from build123d import *

# Parameters (mm, degrees)
SKETCH1_R           = 5.05
BOSS_EXTRUDE1_DEPTH = 20
SKETCH2_R           = 9.25
CUT_EXTRUDE1_DEPTH  = 8
SKETCH4_R           = 7
SKETCH4_R_2         = 4
BOSS_EXTRUDE2_DEPTH = 2
CUT_EXTRUDE2_DEPTH  = 10


with BuildPart() as part:
    # Sketch1 → Boss-Extrude1 (new body)
    with BuildSketch(Plane.XY):
        with BuildLine():
            Line((-3, 10.5), (3, 10.5))
            Line((3, 10.5), (3, 11.618950039))
            ThreePointArc((3, 11.618950039), (8.485281374, 8.485281374), (11.618950039, 3))
            Line((11.618950039, 3), (10.5, 3))
            Line((10.5, 3), (10.5, -3))
            Line((10.5, -3), (11.618950039, -3))
            ThreePointArc((11.618950039, -3), (8.485281374, -8.485281374), (3, -11.618950039))
            Line((3, -11.618950039), (3, -10.5))
            Line((3, -10.5), (-3, -10.5))
            Line((-3, -10.5), (-3, -11.618950039))
            ThreePointArc((-3, -11.618950039), (-8.485281374, -8.485281374), (-11.618950039, -3))
            Line((-11.618950039, -3), (-10.5, -3))
            Line((-10.5, -3), (-10.5, 3))
            Line((-10.5, 3), (-11.618950039, 3))
            ThreePointArc((-11.618950039, 3), (-8.485281374, 8.485281374), (-3, 11.618950039))
            Line((-3, 11.618950039), (-3, 10.5))
        make_face()
        Circle(SKETCH1_R, mode=Mode.SUBTRACT)
    extrude(amount=BOSS_EXTRUDE1_DEPTH)

    # Sketch2 → Cut-Extrude1 (cut)
    with BuildSketch(Plane.XY.offset(20)):
        Circle(SKETCH2_R)
    extrude(amount=-CUT_EXTRUDE1_DEPTH, mode=Mode.SUBTRACT)

    # Cut-Sweep1: sweep along a curve in space
    with BuildLine() as cut_sweep1_path:
        ThreePointArc((9.25, 0, 20), (6.540737726, 6.540737726, 20), (0, 9.25, 20))
        ThreePointArc((0, 9.25, 20), (-6.540737726, 6.540737726, 20), (-9.25, 0, 20))
        ThreePointArc((-9.25, 0, 20), (-6.540737726, -6.540737726, 20), (0, -9.25, 20))
        ThreePointArc((0, -9.25, 20), (6.540737726, -6.540737726, 20), (9.25, 0, 20))
    # Sketch3 → Cut-Sweep1 (sweep, cut)
    with BuildSketch(Plane.XZ.offset(-3)):
        Polygon((10.118950039, 8.968340129), (10.118950039, 11.031659871), (11.618950039, 13.629736082), (11.618950039, 6.370263918), align=None)
    sweep(path=cut_sweep1_path.line, mode=Mode.SUBTRACT)

    # Sketch4 → Boss-Extrude2 (add)
    with BuildSketch(Plane.XY.offset(12)):
        Circle(SKETCH4_R)
        Circle(SKETCH4_R_2, mode=Mode.SUBTRACT)
    extrude(amount=-BOSS_EXTRUDE2_DEPTH)

    # Sketch5 → Cut-Extrude2 (cut)
    with BuildSketch(Plane(origin=(0, 0, 0), x_dir=(-1, 0, 0), z_dir=(0, 0, -1))):
        with BuildLine():
            Line((-11.618950039, 3), (-9.618950039, 3))
            ThreePointArc((-9.618950039, 3), (-8.204736476, 2.414213562), (-7.618950039, 1))
            Line((-7.618950039, 1), (-7.618950039, -1))
            ThreePointArc((-7.618950039, -1), (-8.204736476, -2.414213562), (-9.618950039, -3))
            Line((-9.618950039, -3), (-11.618950039, -3))
            Line((-11.618950039, -3), (-11.618950039, 3))
        make_face()
        with BuildLine():
            Line((-3, -11.618950039), (3, -11.618950039))
            Line((3, -11.618950039), (3, -9.618950039))
            ThreePointArc((3, -9.618950039), (2.414213562, -8.204736476), (1, -7.618950039))
            Line((1, -7.618950039), (-1, -7.618950039))
            ThreePointArc((-1, -7.618950039), (-2.414213562, -8.204736476), (-3, -9.618950039))
            Line((-3, -9.618950039), (-3, -11.618950039))
        make_face()
        with BuildLine():
            Line((3, 11.618950039), (3, 9.618950039))
            ThreePointArc((3, 9.618950039), (2.414213562, 8.204736476), (1, 7.618950039))
            Line((1, 7.618950039), (-1, 7.618950039))
            ThreePointArc((-1, 7.618950039), (-2.414213562, 8.204736476), (-3, 9.618950039))
            Line((-3, 9.618950039), (-3, 11.618950039))
            Line((-3, 11.618950039), (3, 11.618950039))
        make_face()
        with BuildLine():
            Line((11.618950039, -3), (9.618950039, -3))
            ThreePointArc((9.618950039, -3), (8.204736476, -2.414213562), (7.618950039, -1))
            Line((7.618950039, -1), (7.618950039, 1))
            ThreePointArc((7.618950039, 1), (8.204736476, 2.414213562), (9.618950039, 3))
            Line((9.618950039, 3), (11.618950039, 3))
            Line((11.618950039, 3), (11.618950039, -3))
        make_face()
    extrude(amount=-CUT_EXTRUDE2_DEPTH, mode=Mode.SUBTRACT)


solid = part.part
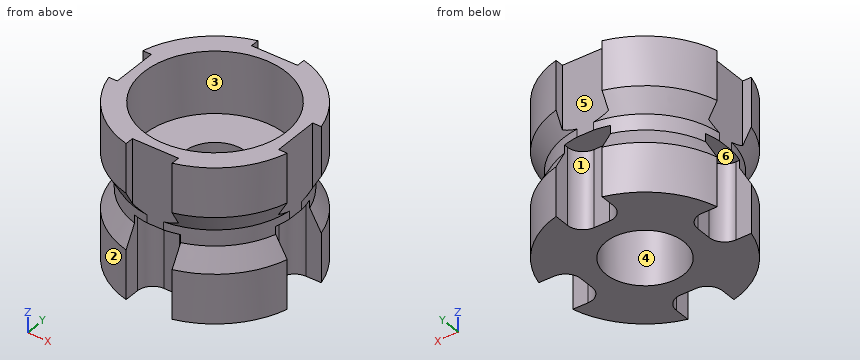
Check sheet for the modelled part. Datum: model origin and axes. Units: mm. Face numbers are marked on the shaded views. A direction names the side the tool comes from. Round coordinates to 2 decimals unless told otherwise and drop trailing zeros. Order: outer loops, then holes, each group sorted by start corner. A loop starts at its lowest first (then second) coordinate and runs counter-clockwise, first axis right, second up.
(1) Cross-section at D-D, the plane z = 10.5. Enter the section's corners in (x, y), and give its area (3 significant figures).
(2) Go/stop test with flat-tipped pins: P1, Ø0.9, axis at x = 11, z = 15.5, coming from the -Y side; P2, Ø1, axis at y = 11, z = 7, coming from the +X side; P3, Ø1, axis at y = -1.5, z = 18, coming from the -X side; P4, Ø8, axis at x = 1.5, y = -4.5, coming from the -Z side. Record where each tip stops, or that it passes through.
(3) Cross-section at A-A, the plane y = 0. Enter the section's corners in (x, z), and give its area (3 significant figures).
(4) Access from +Z, -Z, +X, -X, +Y, -Y to the whole of each face (thin tool, end or side, straight path). Record for the marked faces 4, 5 and 6.
(5) Scan lines: probe 1 along Y at (x, z) = (0, 10.9); probe 2 along Y at (x, z) = (0, 5.5). Record each from-to range of solid material in increasing order.
(6) Draft check along Y on the marked faces 1, 2 and 3. Enter one of: pulls with the +Y half, pulls with the -Y half, needs draft (parallel to the pull), parting line crosses it, or undercut.
(7) Cross-section at C-C, the plane z = 4.5. Enter the section's corners in (x, y), and give its area (3 significant figures).
Check sheet entries:
1. outline: (-10.5, -1.07) arc R10.55 ccw to (-1.07, -10.5) - (1.07, -10.5) arc R10.55 ccw to (10.5, -1.07) - (10.5, 1.07) arc R10.55 ccw to (1.07, 10.5) - (-1.07, 10.5) arc R10.55 ccw to (-10.5, 1.07) - close; hole circle Ø8 at (0, 0)
1. area: 299 mm2
2. P1: stops at y = -5.72
2. P2: stops at x = 5.22
2. P3: stops at x = -10.5
2. P4: stops at z = 0
3. outline: (-10.5, 10) - (-7.62, 10) - (-7.62, 0) - (-5.05, 0) - (-5.05, 10) - (-4, 10) - (-4, 12) - (-9.25, 12) - (-9.25, 20) - (-10.5, 20) - close; (4, 10) - (5.05, 10) - (5.05, 0) - (7.62, 0) - (7.62, 10) - (10.5, 10) - (10.5, 20) - (9.25, 20) - (9.25, 12) - (4, 12) - close
3. area: 97.4 mm2
4. face 4: -Z
4. face 5: +Z, -Z, +Y
4. face 6: -Z, -X
5. probe 1: y = -10.5 to -4, 4 to 10.5
5. probe 2: y = -7.62 to -5.05, 5.05 to 7.62
6. face 1: pulls with the +Y half
6. face 2: pulls with the -Y half
6. face 3: undercut
7. outline: (-11.62, -3) arc R12 ccw to (-3, -11.62) - (-3, -9.62) arc R2 cw to (-1, -7.62) - (1, -7.62) arc R2 cw to (3, -9.62) - (3, -11.62) arc R12 ccw to (11.62, -3) - (9.62, -3) arc R2 cw to (7.62, -1) - (7.62, 1) arc R2 cw to (9.62, 3) - (11.62, 3) arc R12 ccw to (3, 11.62) - (3, 9.62) arc R2 cw to (1, 7.62) - (-1, 7.62) arc R2 cw to (-3, 9.62) - (-3, 11.62) arc R12 ccw to (-11.62, 3) - (-9.62, 3) arc R2 cw to (-7.62, 1) - (-7.62, -1) arc R2 cw to (-9.62, -3) - close; hole circle Ø10.1 at (0, 0)
7. area: 277 mm2
